Answer from the drawing. Dimensions are ordinates in mm from the lowest x, y and z of the part. Give positions to 0.01 mm unless a question says otherwise; leave off trailing zeros. Loops run counter-clockwise (first coordinate to the right, second up) from the corner with the lowest first, then second, coordinate; pieces in that order, holes last. Notation, with made-up numbers: M 0.25,40 L 52.25,40 A31 ccw 52.25,71 Z; hole C -30.75,70 d2. An arc over 180 degrees is marked long. Use a Markdown table: item, result.
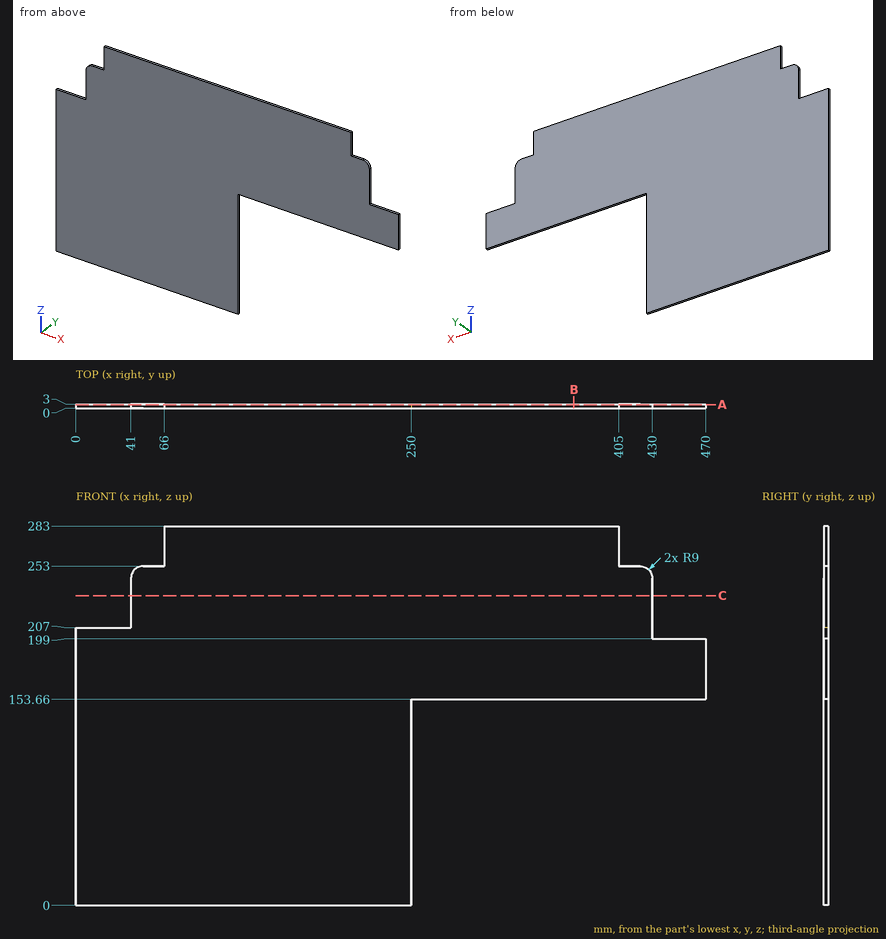
(1) A cutting plane is placed at C-C (z = 231). Write down the section's boundary in (x, y).
Entries:
| item | result |
|---|---|
| outline | M 41,0 L 430,0 L 430,3 L 41,3 Z |
(2) Given P1, Ø1.5, axis at y = 2, z = 234.5, coming from the -X side; P2, Ø1.5, axis at y = 2, z = 262, coming from the -X side; P3, Ø1.5, axis at x = 56, y = 2, coming from the +Z side; P4, Ø8, axis at x = 280.5, z = 146, coming from the -Y side, each flat-ended and moving along its own axis, determine where each tip first touches the part or whether it passes through.
Entries:
| item | result |
|---|---|
| P1 | stops at x = 41 |
| P2 | stops at x = 66 |
| P3 | stops at z = 253 |
| P4 | passes through |
(3) A cutting plane is placed at A-A (y = 2.5). Write down the section's boundary in (x, z).
Entries:
| item | result |
|---|---|
| outline | M 0,0 L 250,0 L 250,153.66 L 470,153.66 L 470,199 L 430,199 L 430,244 A9 ccw 421,253 L 405,253 L 405,283 L 66,283 L 66,253 L 50,253 A9 ccw 41,244 L 41,207 L 0,207 Z |
(4) Consider probe 1 along X at (y, z) = (2.45, 29.5); probe 2 along Z at (x, y) = (396, 2.6); probe 3 along Z at (x, y) = (443, 2). Determine where each line is inside the solid, lowest interval first. Write a range as [from, to].
Entries:
| item | result |
|---|---|
| probe 1 | x = [0, 250] |
| probe 2 | z = [153.66, 283] |
| probe 3 | z = [153.66, 199] |
(5) A cutting plane is placed at B-B (x = 371.5). Write down the section's boundary in (y, z), and give its area (3 significant figures).
Entries:
| item | result |
|---|---|
| outline | M 0,153.66 L 3,153.66 L 3,283 L 0,283 Z |
| area | 388 mm² |
